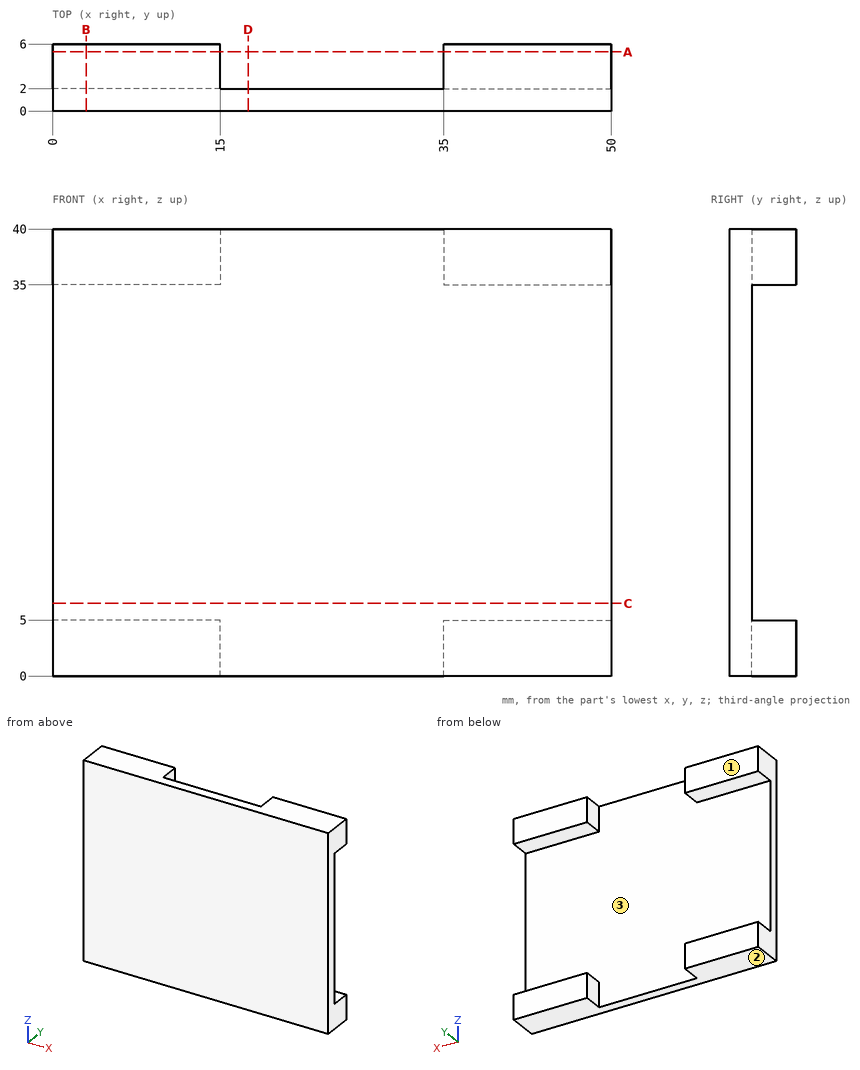
Design review of the part shown in the three views and the two pictorial views. Dimensions are in mm from the part's minimum x, y and z. Give positions to 0.01 mm unless a question says otherwise; leave off trailing zeros. Loops run counter-clockwise (first coordinate to the right, second up) from the corner with the lowest first, then second, coordinate; pieces in that order, holes last. Notation, with made-up numbers: (25.25, -23.5) - (32.25, -23.5) arc R6 cw to (32.25, -14.5) - close; hole circle Ø11 at (45, 29). An arc over 180 degrees is marked (long way). Write item = value, one per line.
1) Clearance check with flat-ended pins moving along their axes: pin 1 Ø1 at (x, y) = (8.5, 2) entering from -Z; pin 2 Ø2 at (x, z) = (29.5, 25.5) entering from +Y. State where each tip first meets the part, or that it passes through.
Result sheet:
pin_1 = 0
pin_2 = 2
2) Take a section at D-D on x = 17.5. State the section outline as (y, z) points.
Result sheet:
outline = (0, 0) - (2, 0) - (2, 40) - (0, 40) - close
3) Take a section at B-B on x = 3. State the section outline as (y, z) points, and give its area (3 significant figures).
Result sheet:
outline = (0, 0) - (6, 0) - (6, 5) - (2, 5) - (2, 35) - (6, 35) - (6, 40) - (0, 40) - close
area = 120 mm2
4) To check wall thickness, follow line 1 (Z direction, x = 10, y = 2.2); line 2 (Y direction, x = 19, z = 28); line 3 (X direction, y = 3, z = 3.5). State the ranges of each line that lie inside material, in increasing order.
Result sheet:
line_1 = 0 to 5, 35 to 40
line_2 = 0 to 2
line_3 = 0 to 15, 35 to 50
5) Take a section at C-C on z = 6.5. State the section outline as (x, y) points, and give its area (3 significant figures).
Result sheet:
outline = (0, 0) - (50, 0) - (50, 2) - (0, 2) - close
area = 100 mm2
6) Draft analysis for pull direction Z (two halves, no side actions). For the marked faces 1, 2 and 3, state which applies: +Z half, -Z half, draft (parallel to the pull), parting line (faces both ways), or undercut.
Result sheet:
face_1 = draft
face_2 = -Z half
face_3 = undercut
7) Take a section at A-A on y = 5.3. State the section outline as (x, z) points.
Result sheet:
outline = (0, 0) - (15, 0) - (15, 5) - (0, 5) - close; (0, 35) - (15, 35) - (15, 40) - (0, 40) - close; (35, 0) - (50, 0) - (50, 5) - (35, 5) - close; (35, 35) - (50, 35) - (50, 40) - (35, 40) - close
